Could you check a few things on this drawing? It's one solid part, dimensions in mm from its lowest x, y, z. Coordinates: 2 decimals unless noted, no trailing zeros. Order: outer loops, then holes, each group sorted by start corner. A loop starts at its lowest first (then second) coordinate and runs counter-clockwise, first axis right, second up.
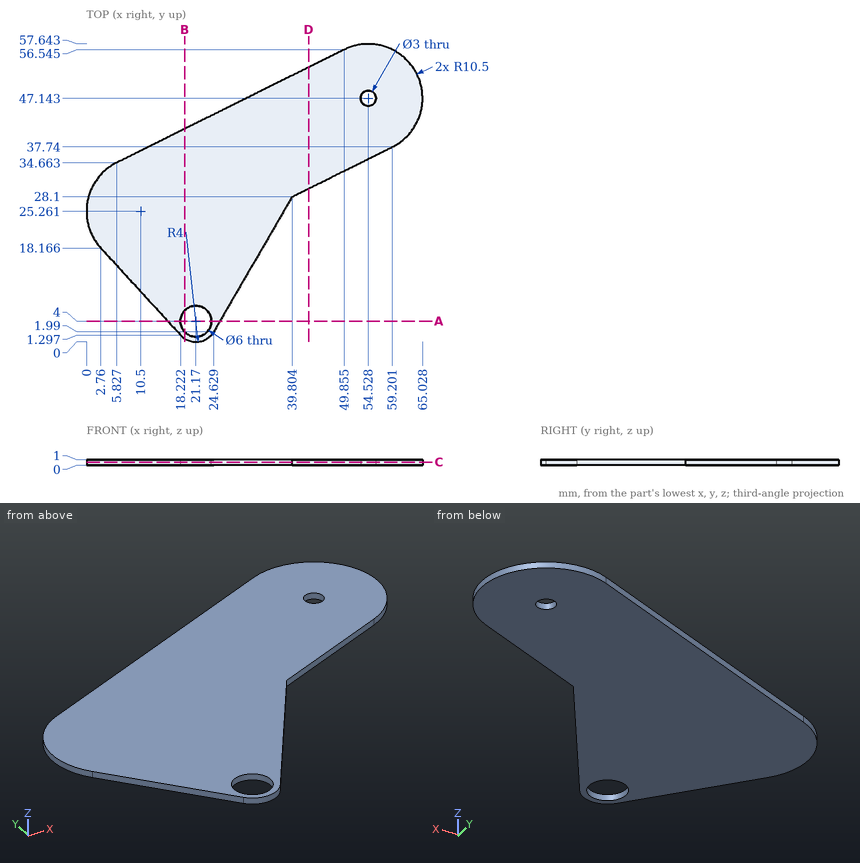
Q1. If we section it at D-D on x = 43: Write out the boundary of the cut face in (y, z).
Q2. I need wall thicknesses on L1, parallel to X at y = 4, z = 0.4 (1 decimal); L2, parallel to Y at x = 54.5, z = 0.85 (1 decimal); L3, parallel to X at y = 46, z = 0.7 (1 decimal). Which ranges of each line are inside material? Lowest first, please.
Q3. If we section it at B-B on x = 19: Write out the boundary of the cut face in (y, z).
Q4. If we section it at C-C on z = 0.55: Write out the boundary of the cut face in (x, y) (1 decimal), then the cut area to 3 significant figures.
Q5. If we section it at A-A on y = 4: Write out the boundary of the cut face in (x, z) (1 decimal).
Reply:
1. outline: (29.69, 0) - (53.14, 0) - (53.14, 1) - (29.69, 1) - close
2. L1: x = 15.7 to 18.2, 24.2 to 25.8
2. L2: y = 35.4 to 45.6, 48.6 to 57.6
2. L3: x = 28.6 to 53.6, 55.5 to 65
3. outline: (0.64, 0) - (1.93, 0) - (1.93, 1) - (0.64, 1) - close; (6.07, 0) - (41.21, 0) - (41.21, 1) - (6.07, 1) - close
4. outline: (2.8, 18.2) - (18.2, 1.3) arc R4 ccw to (24.6, 2) - (39.8, 28.1) - (59.2, 37.7) arc R10.5 ccw to (49.9, 56.5) - (5.8, 34.7) arc R10.5 ccw to start; hole circle Ø6 at (21.2, 4); hole circle Ø3 at (54.5, 47.1)
4. area: 1,700 mm2
5. outline: (15.7, 0) - (18.2, 0) - (18.2, 1) - (15.7, 1) - close; (24.2, 0) - (25.8, 0) - (25.8, 1) - (24.2, 1) - close
